Geometry: final body of the model. Coordinates: model frame, mm. A direction names the side the tool comes from. Coordinates: 2 decimals unless noted, no trailing zeros. Order: outer loops, then holes, each group sorted by start corner. A loop starts at its lowest first (then second) coordinate and runs counter-clockwise, first axis right, second up. Notation, with made-up numbers: (-6, 20) - (31, 20) arc R21 ccw to (31, 57) - close; hole circle Ø2 at (-5.5, 28). An arc over 180 degrees is marked (long way). Use one line per item in the form item = value. Start each with the question number.
```python
from build123d import *

# Parameters (mm, degrees)
SKETCH1_W               = 3
SKETCH1_H               = 80
BOSS_EXTRUDE1_DEPTH     = 50
SKETCH6_W               = 3
SKETCH6_H               = 12
BOSS_EXTRUDE2_DEPTH     = 35
SKETCH14_R              = 18
SKETCH14_R_2            = 15.5
BOSS_EXTRUDE3_DEPTH     = 25
BOSS_EXTRUDE4_DEPTH     = 2.3
CIRPATTERN1_COUNT       = 6
BOSS_EXTRUDE5_START     = -25
BOSS_EXTRUDE5_DEPTH     = 25
BOSS_EXTRUDE6_START     = -25
SKETCH17_R              = 15.5
SKETCH17_R_2            = 13
BOSS_EXTRUDE6_DEPTH     = 19
CUT_EXTRUDE1_DEPTH      = 118.245469157
CUT_EXTRUDE1_DEPTH_BACK = 118.245469157
SKETCH18_W              = 10
SKETCH18_H              = 15


with BuildPart() as part:
    # Sketch1 → Boss-Extrude1 (new body)
    with BuildSketch(Plane(origin=(15.5, 0, 0), x_dir=(0, 0, -1), z_dir=(1, 0, 0))):
        with Locations((0, 52)):
            Rectangle(SKETCH1_W, SKETCH1_H)
    extrude(amount=BOSS_EXTRUDE1_DEPTH)

    # Sketch6 → Boss-Extrude2 (add)
    with BuildSketch(Plane.ZY.offset(-15.5)):
        with Locations((0, 6)):
            Rectangle(SKETCH6_W, SKETCH6_H)
    extrude(amount=-BOSS_EXTRUDE2_DEPTH)

    # Sketch7 → Loft3 section 0
    with BuildSketch(Plane(origin=(50.5, 0, 0), x_dir=(0, 0, -1), z_dir=(1, 0, 0))):
        with BuildLine():
            Line((-1.5, 12), (1.5, 12))
            Line((1.5, 12), (1.5, 0))
            Line((1.5, 0), (-1.5, 0))
            Line((-1.5, 0), (-1.5, 12))
        make_face()
    # Sketch5 → Loft3 section 1
    with BuildSketch(Plane(origin=(65.5, 0, 0), x_dir=(0, 0, -1), z_dir=(1, 0, 0))):
        with BuildLine():
            Line((-1.5, 12), (2.5, 12))
            add(Edge.make_bspline(
                [(2.5, 12), (16.446218703, 4.628977133), (31.5, 0)],
                knots=[0, 0, 0, 1, 1, 1], degree=2))
            Line((31.5, 0), (-31.5, 0))
            add(Edge.make_bspline(
                [(-1.5, 12), (-16.07182757, 4.906260237), (-31.5, 0)],
                knots=[0, 0, 0, 1, 1, 1], degree=2))
        make_face()
    loft()


with BuildPart() as body_2:
    # Mirror3: mirrored copy
    add(part.part.mirror(Plane(origin=(0, 0, 0), x_dir=(0, 0, 1), z_dir=(1, 0, 0))))


with BuildPart() as part_1:
    add(part.part)

    add(body_2.part)  # Boss-Extrude3 merges body 2
    # Sketch14 → Boss-Extrude3 (add)
    with BuildSketch(Plane(origin=(0, 0, 0), x_dir=(1, 0, 0), z_dir=(0, 1, 0))):
        Circle(SKETCH14_R)
        with Locations(Location((0, 0, 0), (0, 0, 180))):
            Circle(SKETCH14_R_2, mode=Mode.SUBTRACT)
    extrude(amount=BOSS_EXTRUDE3_DEPTH)

    # Sketch15 → Boss-Extrude4 (add)
    with BuildSketch(Plane(origin=(0, 25, 0), x_dir=(1, 0, 0), z_dir=(0, 1, 0))):
        Polygon((-1.65, 15.411927199), (-1.65, 14.411927199), (1.65, 14.411927199), (1.65, 15.411927199), (0, 16.251375975), align=None)
    boss_extrude4 = extrude(amount=-BOSS_EXTRUDE4_DEPTH)

    # CirPattern1: Boss-Extrude4 ×6 about axis
    cirpattern1_axis = Axis((0, 0, 0), (0, 1, 0))
    for i in range(1, CIRPATTERN1_COUNT):
        add(boss_extrude4.rotate(cirpattern1_axis, i * 360 / CIRPATTERN1_COUNT))

    # Sketch16 → Boss-Extrude5 (add)
    with BuildSketch(Plane(origin=(0, 25, 0), x_dir=(1, 0, 0), z_dir=(0, 1, 0)).offset(BOSS_EXTRUDE5_START)):
        with BuildLine():
            Line((-18.937391115, 1.5), (-18.937391115, 19.5))
            Line((-18.937391115, 19.5), (18.937391115, 19.5))
            Line((18.937391115, 19.5), (18.937391115, 1.5))
            Line((18.937391115, 1.5), (17.937391115, 1.5))
            ThreePointArc((17.937391115, 1.5), (0, 18), (-17.937391115, 1.5))
            Line((-17.937391115, 1.5), (-18.937391115, 1.5))
        make_face()
    extrude(amount=BOSS_EXTRUDE5_DEPTH)

    # Sketch17 → Boss-Extrude6 (add)
    with BuildSketch(Plane(origin=(0, 25, 0), x_dir=(1, 0, 0), z_dir=(0, 1, 0)).offset(BOSS_EXTRUDE6_START)):
        with Locations(Location((0, 0, 0), (0, 0, 96.110806636))):
            Circle(SKETCH17_R)
        with Locations(Location((0, 0, 0), (0, 0, 270))):
            Circle(SKETCH17_R_2, mode=Mode.SUBTRACT)
    extrude(amount=BOSS_EXTRUDE6_DEPTH)

    # Sketch18 → Cut-Extrude1 (cut, two sides: drawn at the far end of the back side and taken through both)
    with BuildSketch(Plane(origin=(0, 0, 0), x_dir=(0, 0, -1), z_dir=(1, 0, 0)).offset(-CUT_EXTRUDE1_DEPTH_BACK)):
        with Locations((-6.5, 17.5)):
            Rectangle(SKETCH18_W, SKETCH18_H)
    extrude(amount=CUT_EXTRUDE1_DEPTH + CUT_EXTRUDE1_DEPTH_BACK, mode=Mode.SUBTRACT)


solid = part_1.part
```
(1) Cut plane C-C on y = 62. Return the cut outline in (x, z).
(2) Cut plane A-A on y = 16.5. Return the cut outline in (x, z), plus the area to 3 significant figures.
(3) Set-up query: faces 4 (the cylindrical face through (0, 10, 18)), 5 (the flat face through (60, 10, 3)), 6 (the cylindrical face through (0.362, 21.958, -15.496)), 7 (the flat face through (-11, 16, 11.5)), 8 (the flat face through (0, 12, -19.5)). Return all of +Z, -Z, +X, -X, +Y, -Y with unobstructed straight access to the full face (end or side cutting, diameter ignored); none if empty.
(4) Cut plane B-B on x = 0. Return the cut outline in (y, z), plus the area to 3 significant figures.
(5) Draft query along X for faces 1 (the flat face through (-65.5, 25, 0)), 2 (the flat face through (-13, 10, 7)), 3 (the flat face through (-15.5, 59, 0)). Return one class per face: released by +X, released by -X, zero draft, split by the parting line, or undercut.
(6) Contact query for flat-ended pins moving along their axis: pin 1 Ø0.8 at (x, z) = (-13, -6.5) entering from -Y; pin 2 Ø8 at (x, y) = (26, 58.5) entering from -Z; pin 3 Ø5 at (x, z) = (-3.5, 14) entering from +Y; pin 4 Ø0.5 at (y, z) = (23.5, 14.5) entering from -X. Output: stop coordinate, or through.
(7) Cut plane D-D on x = 24.5. Return the cut outline in (y, z), plus the area to 3 significant figures.
(8) Material intervals for L1, parallel to Z at x = 0, y = 22.4; L2, parallel to Z at x = 0, y = 10.25; L3, parallel to X at y = 22.75, z = 0, sorted ascending. Write a range as from..to.
Check sheet entries:
q1.outline = (-65.5, -1.5) - (-15.5, -1.5) - (-15.5, 1.5) - (-65.5, 1.5) - close; (15.5, -1.5) - (65.5, -1.5) - (65.5, 1.5) - (15.5, 1.5) - close
q2.outline = (-65.5, -1.5) - (-18.94, -1.5) - (-18.94, -19.5) - (18.94, -19.5) - (18.94, -1.5) - (65.5, -1.5) - (65.5, 1.5) - (12.91, 1.5) arc R13 cw (long way) to (-12.91, 1.5) - (-65.5, 1.5) - close; (-13.85, 11.5) - (-6.06, 11.5) arc R13 cw to (6.06, 11.5) - (13.85, 11.5) arc R18 ccw to start
q2.area = 883 mm^2
q3.face_4 = +Z, +Y, -Y
q3.face_5 = +Z, +X, -X, +Y
q3.face_6 = none
q3.face_7 = +X, -X, +Y
q3.face_8 = -Z, +Y, -Y
q4.outline = (0, -19.5) - (25, -19.5) - (25, -14.41) - (22.7, -14.41) - (22.7, -15.5) - (19, -15.5) - (19, -13) - (0, -13) - close; (0, 13) - (19, 13) - (19, 15.5) - (22.7, 15.5) - (22.7, 14.41) - (25, 14.41) - (25, 18) - (0, 18) - close
q4.area = 263 mm^2
q5.face_1 = released by -X
q5.face_2 = zero draft
q5.face_3 = undercut
q6.pin_1 = 0
q6.pin_2 = -1.5
q6.pin_3 = 25
q6.pin_4 = -11
q7.outline = (0, -1.5) - (92, -1.5) - (92, 1.5) - (0, 1.5) - close
q7.area = 276 mm^2
q8.L1 = -19.5..-15.5, 15.5..18
q8.L2 = -19.5..-13, 13..18
q8.L3 = -65.5..-15.5, 15.5..65.5
